Could you check a few things on this model? Use its own coordinates, in mm. Face numbers are marked on the shaded views. Round coordinates to 2 decimals unless told otherwise and drop trailing zeros. Order: outer loops, then holes, each group sorted by start corner. A loop starts at its lowest first (then second) coordinate and runs counter-clockwise, first axis right, second up.
```python
from build123d import *

# Parameters (mm, degrees)
ESQUISSE1_W             = 50
ESQUISSE1_H             = 15
BOSS_EXTRU_1_DEPTH      = 7.5
ESQUISSE3_R             = 3
ENL_V_MAT_EXTRU_2_DEPTH = 31.103986447
ESQUISSE4_W             = 15
ESQUISSE4_H             = 3
ENL_V_MAT_EXTRU_3_DEPTH = 15
ESQUISSE5_W             = 15
ESQUISSE5_H             = 3
ENL_V_MAT_EXTRU_4_DEPTH = 15


with BuildPart() as part:
    # Esquisse1 → Boss.-Extru.1 (new, symmetric)
    with BuildSketch(Plane(origin=(0, 0, 0), x_dir=(0, 0, -1), z_dir=(1, 0, 0))):
        Rectangle(ESQUISSE1_W, ESQUISSE1_H)
    extrude(amount=BOSS_EXTRU_1_DEPTH, both=True)

    # Esquisse3 → Enlèv. mat.-Extru.2 (cut, through all)
    with BuildSketch(Plane(origin=(0, 7.5, 0), x_dir=(1, 0, 0), z_dir=(0, 1, 0))):
        with Locations(Location((0, 17, 0), (0, 0, 270))):
            Circle(ESQUISSE3_R)
        with Locations(Location((0, -17, 0), (0, 0, 270))):
            Circle(ESQUISSE3_R)
    extrude(amount=-ENL_V_MAT_EXTRU_2_DEPTH, mode=Mode.SUBTRACT)

    # Esquisse4 → Enlèv. mat.-Extru.3 (cut)
    with BuildSketch(Plane.XY.offset(25)):
        Rectangle(ESQUISSE4_W, ESQUISSE4_H)
    extrude(amount=-ENL_V_MAT_EXTRU_3_DEPTH, mode=Mode.SUBTRACT)

    # Esquisse5 → Enlèv. mat.-Extru.4 (cut)
    with BuildSketch(Plane(origin=(0, 0, -25), x_dir=(-1, 0, 0), z_dir=(0, 0, -1))):
        Rectangle(ESQUISSE5_W, ESQUISSE5_H)
    extrude(amount=-ENL_V_MAT_EXTRU_4_DEPTH, mode=Mode.SUBTRACT)


solid = part.part
```
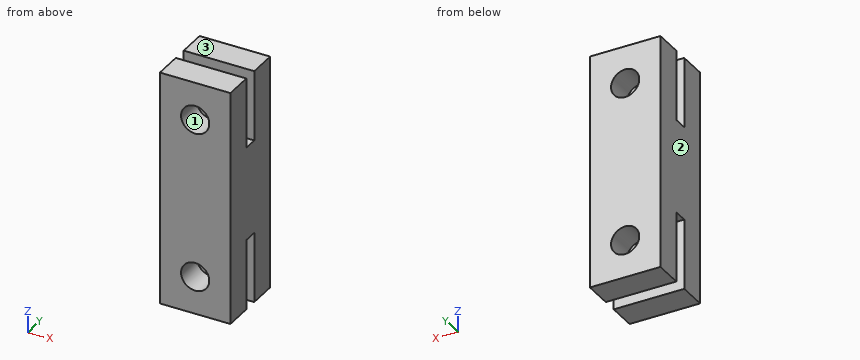
Q1. We'd pull the mould along X, two halves only. Please class the marked faces 1, 2 and 3: released by +X, released by -X, zero draft, split by the parting line, or undercut.
Q2. For P1, Ø1.5, axis at x = -0.5, y = 0, coming from the +Z side; P2, Ø1.5, axis at x = 1, y = 0.5, coming from the -Z side, each with a flat end and sliding along its axis, tell me the tip position at first contact or that it passes through.
Q3. Imagine slicing it at D-D, the plane y = -4.5. Please give me the cut outline in (x, z).
Q4. I need wall thicknesses on L1, parallel to X at y = 5.25, z = -17; L2, parallel to Y at x = -2.75, z = -12; L3, parallel to Z at x = 1.5, y = 5.25. Which ranges of each line are inside material? Lowest first, please.
Q5. Imagine slicing it at C-C, the plane z = 11. Please give me the cut outline in (x, y), then the cut area to 3 significant figures.
Q6. Imagine slicing it at B-B, the plane x = 0. Please give me the cut outline in (y, z).
Q7. Imagine slicing it at A-A, the plane z = 17. Please give me the cut outline in (x, y), then the cut area to 3 significant figures.
Filled in:
1. face 1: undercut
1. face 2: released by -X
1. face 3: zero draft
2. P1: stops at z = 10
2. P2: stops at z = -10
3. outline: (-7.5, -25) - (7.5, -25) - (7.5, 25) - (-7.5, 25) - close; hole circle Ø6 at (0, -17); hole circle Ø6 at (0, 17)
4. L1: x = -7.5 to -3, 3 to 7.5
4. L2: y = -7.5 to -1.5, 1.5 to 7.5
4. L3: z = -25 to -19.6, -14.4 to 14.4, 19.6 to 25
5. outline: (-7.5, -7.5) - (7.5, -7.5) - (7.5, -1.5) - (-7.5, -1.5) - close; (-7.5, 1.5) - (7.5, 1.5) - (7.5, 7.5) - (-7.5, 7.5) - close
5. area: 180 mm2
6. outline: (-7.5, -25) - (-1.5, -25) - (-1.5, -20) - (-7.5, -20) - close; (-7.5, -14) - (-1.5, -14) - (-1.5, -10) - (1.5, -10) - (1.5, -14) - (7.5, -14) - (7.5, 14) - (1.5, 14) - (1.5, 10) - (-1.5, 10) - (-1.5, 14) - (-7.5, 14) - close; (-7.5, 20) - (-1.5, 20) - (-1.5, 25) - (-7.5, 25) - close; (1.5, -25) - (7.5, -25) - (7.5, -20) - (1.5, -20) - close; (1.5, 20) - (7.5, 20) - (7.5, 25) - (1.5, 25) - close
7. outline: (-7.5, -7.5) - (-3, -7.5) - (-3, -1.5) - (-7.5, -1.5) - close; (-7.5, 1.5) - (-3, 1.5) - (-3, 7.5) - (-7.5, 7.5) - close; (3, -7.5) - (7.5, -7.5) - (7.5, -1.5) - (3, -1.5) - close; (3, 1.5) - (7.5, 1.5) - (7.5, 7.5) - (3, 7.5) - close
7. area: 108 mm2
